from build123d import *

# Parameters (mm, degrees)
BOSS_EXTRUDE2_DEPTH = 2
SKETCH3_W           = 80
SKETCH3_H           = 8
BOSS_EXTRUDE3_DEPTH = 3
SKETCH4_R           = 1.5
BOSS_EXTRUDE4_DEPTH = 7
SKETCH12_R          = 1.5
BOSS_EXTRUDE6_DEPTH = 4
SKETCH14_W          = 10
SKETCH14_H          = 8
CUT_EXTRUDE1_DEPTH  = 3
SKETCH15_R          = 1.5
BOSS_EXTRUDE7_DEPTH = 7
FILLET1_R           = 4


with BuildPart() as part:
    # Sketch1 → Boss-Extrude2 (new body)
    with BuildSketch(Plane(origin=(0, 0, 0), x_dir=(1, 0, 0), z_dir=(0, 1, 0))):
        with BuildLine():
            Line((-25, -4), (65, -4))
            ThreePointArc((65, -4), (69, 0), (65, 4))
            Line((65, 4), (-25, 4))
            Line((-25, 4), (-25, -4))
        make_face()
    extrude(amount=BOSS_EXTRUDE2_DEPTH)

    # Sketch3 → Boss-Extrude3 (add)
    with BuildSketch(Plane(origin=(0, 2, 0), x_dir=(1, 0, 0), z_dir=(0, 1, 0))):
        with Locations((15, 0)):
            Rectangle(SKETCH3_W, SKETCH3_H)
    extrude(amount=BOSS_EXTRUDE3_DEPTH)

    # Sketch4 → Boss-Extrude4 (add)
    with BuildSketch(Plane(origin=(0, 2, 0), x_dir=(1, 0, 0), z_dir=(0, 1, 0))):
        with Locations(Location((65, 0, 0), (0, 0, 270))):
            Circle(SKETCH4_R)
    extrude(amount=BOSS_EXTRUDE4_DEPTH)

    # Sketch12 → Boss-Extrude6 (add)
    with BuildSketch(Plane(origin=(0, 5, 0), x_dir=(1, 0, 0), z_dir=(0, 1, 0))):
        with Locations(Location((47, 0, 0), (0, 0, 270))):
            Circle(SKETCH12_R)
        with Locations(Location((27, 0, 0), (0, 0, 270))):
            Circle(SKETCH12_R)
        with Locations(Location((7, 0, 0), (0, 0, 270))):
            Circle(SKETCH12_R)
    extrude(amount=BOSS_EXTRUDE6_DEPTH)

    # Sketch14 → Cut-Extrude1 (cut)
    with BuildSketch(Plane(origin=(0, 5, 0), x_dir=(1, 0, 0), z_dir=(0, 1, 0))):
        with Locations((-20, 0)):
            Rectangle(SKETCH14_W, SKETCH14_H)
    extrude(amount=-CUT_EXTRUDE1_DEPTH, mode=Mode.SUBTRACT)

    # Sketch15 → Boss-Extrude7 (add)
    with BuildSketch(Plane(origin=(0, 2, 0), x_dir=(1, 0, 0), z_dir=(0, 1, 0))):
        with Locations(Location((-22, 0, 0), (0, 0, 270))):
            Circle(SKETCH15_R)
    extrude(amount=BOSS_EXTRUDE7_DEPTH)

    # Fillet1
    fillet1_edges = [part.edges().sort_by_distance(p)[0] for p in [
        (-25, 1, -4),
        (-25, 1, 4),
    ]]
    fillet(fillet1_edges, radius=FILLET1_R - 0.0001)  # a hair under: the kernel refuses the full size


solid = part.part
Verification items for the finished model (mm, model axes). A direction names the side the tool comes from. Give positions to 0.01 mm unless a question says otherwise; leave off trailing zeros. Loops run counter-clockwise (first coordinate to the right, second up) from the corner with the lowest first, then second, coordinate; pieces in that order, holes last.
1. Release check for a two-part mould opening along X. For faces 1 (the cylindrical face through (-23.859, 1.014, 2.797)), 2 (the flat face through (62, 2, 0)), 3 (the flat face through (65, 9, 0)) record: +X half, -X half, draft (parallel to the pull), parting line (faces both ways), or undercut.
Derived:
face 1: -X half
face 2: undercut
face 3: draft
2. Cross-section at A-A on y = 4. Record the cut outline in (x, z), and give its area (3 significant figures).
Derived:
outline: circle Ø3 at (-22, 0); (-15, -4) - (55, -4) - (55, 4) - (-15, 4) - close; circle Ø3 at (65, 0)
area: 574 mm2
3. Material ranges on probe 1 along X at (y, z) = (3.25, -0.25); probe 2 along X at (y, z) = (3, -0.5); probe 3 along Y at (x, z) = (39.5, 3.75), recorded low to high.
Derived:
probe 1: x = -23.48 to -20.52, -15 to 55, 63.52 to 66.48
probe 2: x = -23.41 to -20.59, -15 to 55, 63.59 to 66.41
probe 3: y = 0 to 5
4. Go/stop test with flat-tipped pins: P1, Ø4, axis at x = 29.5, z = 1, coming from the +Y side; P2, Ø0.9, axis at y = 3.5, z = -1, coming from the +X side; P3, Ø4, axis at y = 5, z = -2, coming from the -X side; P4, Ø1.5, axis at y = 1.5, z = -3, coming from the +X side. Record where each tip stops, or that it passes through.
Derived:
P1: stops at y = 9
P2: stops at x = 66.4
P3: stops at x = -23.5
P4: stops at x = 68.31
5. Tool access check on faces 4 (the flat face through (55, 3, 0)), 5 (the flat face through (27, 9, 0)), 6 (the cylindrical face through (28.487, 6.972, -0.195)). Record the directions out of +Z, -Z, +X, -X, +Y, -Y that give a thin tool (end or side, any length) a straight path to the whole face; none if there is none.
Derived:
face 4: +Z, -Z, +Y
face 5: +Z, -Z, +X, -X, +Y
face 6: +Y
6. Cross-section at D-D on z = 2.5. Record the cut outline in (x, y), and give its area (3 significant figures).
Derived:
outline: (-24.12, 0) - (68.12, 0) - (68.12, 2) - (55, 2) - (55, 5) - (-15, 5) - (-15, 2) - (-24.12, 2) - close
area: 394 mm2
7. Cross-section at C-C on y = 8. Record the cut outline in (x, z).
Derived:
outline: circle Ø3 at (-22, 0); circle Ø3 at (7, 0); circle Ø3 at (27, 0); circle Ø3 at (47, 0); circle Ø3 at (65, 0)
8. Cross-section at B-B on x = 7. Record the cut outline in (y, z).
Derived:
outline: (0, -4) - (5, -4) - (5, -1.5) - (9, -1.5) - (9, 1.5) - (5, 1.5) - (5, 4) - (0, 4) - close
